```python
from build123d import *

# Parameters (mm, degrees)
F1_DEPTH = 6.096
F2_DEPTH = 5.08
F0_R     = 1.5875
F3_DEPTH = 3.175
F4_DEPTH = 5.08


# Not quite as in the source:
# - a feature names something its author has since deleted; it is built from what else it names


with BuildPart() as f1:
    # F0 (on Top) → F1 (new body)
    with BuildSketch(Plane.XY):
        Polygon((-24.1886169598, 3.2886979016), (-29.4082708062, 3.2886979016), (-29.4082708062, -20.4897223923), (-23.292648052, -20.4897223923), (-23.292648052, -14.4124455645), (-23.292648052, -10.3212194436), (-20.7735943805, -20.2349212979), (-20.7088498843, -20.4897223923), (-20.6143816365, -20.4897223923), (-16.92762383, -20.4897223923), (-15.8206042222, -20.4897223923), (-15.8206042222, -9.7183147231), (-15.8206042222, -6.9649312645), (-15.8206042222, 3.2886979016), (-16.92762383, 3.2886979016), (-20.6143816365, 3.2886979016), (-21.6202178109, 3.2886979016), (-21.6202178109, 1.5303949543), (-21.6202178109, -6.8192024151), (-22.9411163325, -1.6208240435), align=None)
    extrude(amount=F1_DEPTH)



with BuildPart() as f1b:
    # F0 (on Top) → F1, piece 2 (new body)
    with BuildSketch(Plane.XY):
        Polygon((-11.8259407802, 3.2886979016), (-13.0638151335, -6.9649312645), (-13.3962186866, -9.7183147231), (-14.6966021007, -20.4897223923), (-9.4239554059, -20.4897223923), (-9.0138624712, -16.2260920352), (-6.6118787134, -16.2260920352), (-6.0260297393, -20.4897223923), (0, -20.4897223923), (-1.6947368922, -9.7183147231), (-2.1279449434, -6.9649312645), (-3.7412163152, 3.2886979016), align=None)
        Polygon((-8.9032554867, -11.7976386267), (-7.9436938241, -2.1282115334), (-6.6930804921, -11.7976386267), align=None, mode=Mode.SUBTRACT)
    extrude(amount=F1_DEPTH)


with BuildPart() as f1c:
    # F0 (on Top) → F1, piece 3 (new body)
    with BuildSketch(Plane.XY):
        Polygon((16.3027588278, 3.2886979016), (13.1864075148, 3.2886979016), (7.2406129912, 3.2886979016), (5.4566214701, -14.5271265076), (2.6535398471, 3.2886979016), (-1.9227857701, 3.2886979016), (-0.5595875609, -6.9649312645), (-0.1935310809, -9.7183147231), (1.23850468, -20.4897223923), (9.7333230228, -20.4897223923), (12.1938914085, -1.1697572338), (15.6504033197, -10.3675947497), (15.6504033197, -16.4159582139), (15.6504033197, -19.8583583692), (17.259035404, -19.8583583692), (21.3917291938, -19.8583583692), (21.3917291938, -10.3090095828), (26.0736756027, 3.2886979016), (19.7453610599, 3.2886979016), (19.0404757801, -1.1567947134), (18.4624816288, -4.8020243761), align=None)
    extrude(amount=F1_DEPTH)


with BuildPart() as f1_1:
    add(f1.part)

    add(f1c.part)  # F2 merges F1c
    # F0 (on Top) → F2 (join)
    with BuildSketch(Plane.XY):
        with BuildLine():
            ThreePointArc((-6.4941192245, 13.1090595505), (-14.544099093, 9.6221382111), (-20.6143816365, 3.2886979016))
            Line((-20.6143816365, 3.2886979016), (-16.92762383, 3.2886979016))
            ThreePointArc((-16.92762383, 3.2886979016), (-1.8706081576, 10.5845610899), (13.1864075148, 3.2886979016))
            Line((13.1864075148, 3.2886979016), (16.3027588278, 3.2886979016))
            Line((16.3027588278, 3.2886979016), (18.4624816288, -4.8020243761))
            Line((18.4624816288, -4.8020243761), (19.0404757801, -1.1567947134))
            ThreePointArc((19.0404757801, -1.1567947134), (12.7148241923, 8.1311202307), (2.6507858926, 13.130556711))
            ThreePointArc((2.6507858926, 13.130556711), (-1.9227857701, 13.595875741), (-6.4941192245, 13.1090595505))
        make_face()
        with BuildLine():
            ThreePointArc((-21.6202178109, 1.5303949543), (-22.3413934423, -0.0197598322), (-22.9411163325, -1.6208240435))
            Line((-22.9411163325, -1.6208240435), (-21.6202178109, -6.8192024151))
            Line((-21.6202178109, -6.8192024151), (-21.6202178109, 1.5303949543))
        make_face()
        with BuildLine():
            Line((-23.292648052, -10.3212194436), (-23.292648052, -14.4124455645))
            ThreePointArc((-23.292648052, -14.4124455645), (-22.2422118931, -17.4141450598), (-20.7735943805, -20.2349212979))
            Line((-20.7735943805, -20.2349212979), (-23.292648052, -10.3212194436))
        make_face()
        with BuildLine():
            Line((-16.92762383, -20.4897223923), (-20.6143816365, -20.4897223923))
            ThreePointArc((-20.6143816365, -20.4897223923), (-1.5006364525, -30.7938779901), (17.259035404, -19.8583583692))
            Line((17.259035404, -19.8583583692), (15.6504033197, -19.8583583692))
            Line((15.6504033197, -19.8583583692), (15.6504033197, -16.4159582139))
            ThreePointArc((15.6504033197, -16.4159582139), (0.5098765571, -27.6373274044), (-16.92762383, -20.4897223923))
        make_face()
    extrude(amount=F2_DEPTH)

    # F0 (on Top) → F3 (join)
    with BuildSketch(Plane.XY):
        with BuildLine():
            ThreePointArc((2.6507858926, 13.130556711), (-1.933592452, 18.1930447362), (-6.4941192245, 13.1090595505))
            ThreePointArc((-6.4941192245, 13.1090595505), (-1.9227857701, 13.595875741), (2.6507858926, 13.130556711))
        make_face()
        with Locations((-1.9227857701, 16.0606782883)):
            Circle(F0_R, mode=Mode.SUBTRACT)
    extrude(amount=F3_DEPTH)


    add(f1b.part)  # F4 merges F1b
    # F0 (on Top) → F4 (join)
    with BuildSketch(Plane.XY):
        Polygon((-13.0638151335, -6.9649312645), (-15.8206042222, -6.9649312645), (-15.8206042222, -9.7183147231), (-13.3962186866, -9.7183147231), align=None)
        Polygon((-0.5595875609, -6.9649312645), (-2.1279449434, -6.9649312645), (-1.6947368922, -9.7183147231), (-0.1935310809, -9.7183147231), align=None)
    extrude(amount=F4_DEPTH)


solid = f1_1.part
```
For this review, take the finished solid that the model builds, in its own axes (mm). A direction names the side the tool comes from. Coordinates: 2 decimals unless noted, no trailing zeros. Write each loop counter-clockwise with the first axis right and the second up, starting at its lowest first coordinate (ties: lowest second). Pieces come first, ordered by that corner, then holes. Notation, with made-up numbers: (36, -25) - (81, -25) arc R18 ccw to (81, 6) - close; hole circle Ø1 at (72, 77.25). An arc over 180 degrees is marked (long way). Put each result on its own line as item: value.
1. Add section B-B, the plane x = 6.5. Give the boundary of the cut face in (y, z).
Values found:
outline: (-29.16, 0) - (-25.86, 0) - (-25.86, 5.08) - (-29.16, 5.08) - close; (-20.49, 0) - (-4.11, 0) - (-4.11, 6.1) - (-20.49, 6.1) - close; (8.66, 0) - (11.96, 0) - (11.96, 5.08) - (8.66, 5.08) - close
2. Machinability: for faces 4 (the flat face through (-1, -9.718, 3)), 5 (the flat face through (-26, -20.49, 3)), 6 (the flat face through (-22.4, -15.3, 5.08)), 7 (the flat face through (-1, -8, 5.08)), which of the approach directions +Z, -Z, +X, -X, +Y, -Y give a long, thin tool a straight path to every point of the face, cutting with its end or side? Answer none if there is none.
Values found:
face 4: +Z, -Z
face 5: +Z, -Z, -X, -Y
face 6: +Z, -Y
face 7: +Z
3. Add section A-A, the plane y = 4. Give the boundary of the cut face in (x, z), then the cut area to 3 significant figures.
Values found:
outline: (-20.14, 0) - (-16.34, 0) - (-16.34, 5.08) - (-20.14, 5.08) - close; (12.6, 0) - (16.4, 0) - (16.4, 5.08) - (12.6, 5.08) - close
area: 38.7 mm²
4. For pin 1 (1.9 mm diameter, centred on x = -1.92, y = 16.06, fed in from -Z); pin 2 (1.7 mm diameter, centred on x = -1, z = 3, fed in from -Y); pin 3 (3 mm diameter, centred on x = 14, z = 4.5, fed in from +Y); pin 4 (0.5 mm diameter, centred on x = -1, z = 3, fed in from +Y), all flat-tipped, find the tip position at first contact; note any pin that passes through.
Values found:
pin 1: through
pin 2: y = -30.8
pin 3: y = 8.32
pin 4: y = 18.14
5. Add section D-D, the plane x = -5. Give the boundary of the cut face in (y, z) (3 decimals).
Values found:
outline: (-30.575, 0) - (-27.529, 0) - (-27.529, 5.08) - (-30.575, 5.08) - close; (-20.49, 0) - (3.289, 0) - (3.289, 6.096) - (-20.49, 6.096) - close; (10.328, 0) - (17.011, 0) - (17.011, 3.175) - (13.374, 3.175) - (13.374, 5.08) - (10.328, 5.08) - close
6. Add section C-C, the plane y = -11. Give the boundary of the cut face in (x, z), then the cut area to 3 significant figures.
Values found:
outline: (-29.41, 0) - (-15.82, 0) - (-15.82, 6.1) - (-23.12, 6.1) - (-23.12, 5.08) - (-23.29, 5.08) - (-23.29, 6.1) - (-29.41, 6.1) - close; (-13.55, 0) - (-8.82, 0) - (-8.82, 6.1) - (-13.55, 6.1) - close; (-6.8, 0) - (-1.49, 0) - (-1.49, 6.1) - (-6.8, 6.1) - close; (-0.02, 0) - (4.9, 0) - (4.9, 6.1) - (-0.02, 6.1) - close; (5.81, 0) - (10.94, 0) - (10.94, 6.1) - (5.81, 6.1) - close; (15.65, 0) - (21.39, 0) - (21.39, 6.1) - (15.65, 6.1) - close
area: 240 mm²
7. Mouldability with a two-part tool opening along X and no side actions: class faces 1 (the flat face through (-21.62, 2, 4)), 2 (the cylindrical face through (-1.826, 18.192, 1.565)), 3 (the flat face through (9, -8, 6.096)) as released by +X, released by -X, zero draft, split by the parting line, or undercut.
Values found:
face 1: undercut
face 2: split by the parting line
face 3: zero draft
8. Wall thickness on probe 1 along X at (y, z) = (0.5, 3.25); probe 2 along X at (y, z) = (-16, 4.25); probe 3 along X at (y, z) = (-17, 5.75): over which ranges is each line inside the solid? List them lowest first.
Values found:
probe 1: -29.41 to -23.48, -22.12 to -15.82, -12.16 to -3.3, -1.55 to 3.09, 6.96 to 18.37, 19.3 to 25.11
probe 2: -29.41 to -23.29, -22.8 to -15.82, -14.15 to -0.71, 0.64 to 10.31, 15.65 to 21.39
probe 3: -29.41 to -23.29, -21.6 to -15.82, -14.28 to -9.09, -6.51 to -0.55, 0.77 to 10.18, 15.65 to 21.39
